Source: CAD feature listing. Evaluate the final solid. Frame: model axes, mm. Coordinates: 2 decimals unless noted, no trailing zeros. Loops run counter-clockwise (first coordinate to the right, second up) from the corner with the lowest first, then second, coordinate; pieces in that order, holes last.
Item 1: Section query B-B, the plane z = -6.4. Return the cut outline in (x, y) (3 decimals), then the cut area to 3 significant figures.
Item 2: Line query: probe 1 along Z at (x, y) = (41.6, 2.45) (3 decimals); probe 2 along Z at (x, y) = (35.2, 0.8) (3 decimals); probe 3 along X at (y, z) = (2, 14.4) (3 decimals). Output: solid intervals per line, ascending.
Item 3: Pin query (flat end, axial travel): pin 1 Ø2.5 at (x, z) = (6.4, 35.2) entering from -Y. Return the tip coordinate at first contact, or that it passes through.
Item 4: Section query D-D, the plane y = 2.5. State how many separate pieces and enclosed holes the cut face has, then the cut area to 3 significant figures.
Item 5: Section query A-A, the plane x = 20.8. Return the cut outline in (y, z) (3 decimals).
Item 6: Section query C-C, the plane x = 6.4. Return the cut outline in (y, z) (3 decimals), then the cut area to 3 significant figures.
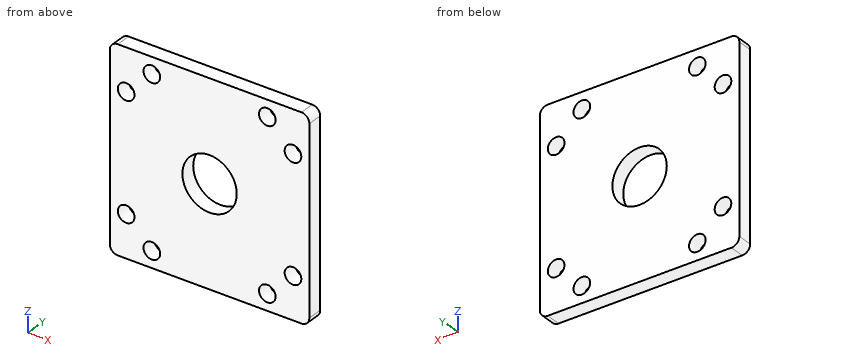
Autodesk Inventor part; units mm, degrees
ref_plane "YZ Plane" through (0, 0, 0) normal (1, 0, 0) x (0, 1, 0)
ref_plane "XZ Plane" through (0, 0, 0) normal (0, 1, 0) x (-1, 0, 0)
ref_plane "XY Plane" through (0, 0, 0) normal (0, 0, 1) x (1, 0, 0)
sketch "Sketch1" plane through (0, 0, 0) normal (0, 1, 0) x (-1, 0, 0)
  circle A0 centre (-20.8, 14.4) radius 6.7838
  circle A1 centre (-42.7, -7.5) radius 1.875
  circle A2 centre (1.1, 36.3) radius 1.875
  circle A3 centre (1.1, -7.5) radius 1.875
  circle A4 centre (-42.7, 36.3) radius 1.875
  circle A5 centre (-6.4, 35.2) radius 2.0734
  circle A6 centre (-35.2, -6.4) radius 2.0734
  circle A7 centre (-6.4, -6.4) radius 2.0734
  circle A8 centre (0, 0) radius 2.0734
  line L0 (-37.85, 31.45) -> (-37.85, -2.65)
  line L1 (-3.75, 31.45) -> (-37.85, 31.45)
  line L2 (-3.75, -2.65) -> (-3.75, 31.45)
  line L3 (-37.85, -2.65) -> (-3.75, -2.65)
  circle A9 centre (0, 28.8) radius 2.0734
  circle A10 centre (-35.2, 35.2) radius 2.0734
  circle A11 centre (-41.6, 0) radius 2.0734
  circle A12 centre (-41.6, 28.8) radius 2.0734
  line L4 (-43.7, 39.275) -> (2.1, 39.275)
  arc A13 (-43.7, 39.275) -> (-45.675, 37.3) centre (-43.7, 37.3) ccw
  line L5 (-45.675, -8.5) -> (-45.675, 37.3)
  arc A14 (-45.675, -8.5) -> (-43.7, -10.475) centre (-43.7, -8.5) ccw
  line L6 (2.1, -10.475) -> (-43.7, -10.475)
  arc A15 (2.1, -10.475) -> (4.075, -8.5) centre (2.1, -8.5) ccw
  line L7 (4.075, 37.3) -> (4.075, -8.5)
  arc A16 (4.075, 37.3) -> (2.1, 39.275) centre (2.1, 37.3) ccw
  line L8 (-3.75, 14.4) -> (-37.85, 14.4)
  dimension "d36" = 13.5675
extrude "Extrusion1" add sketch "Sketch1" along normal blind 3.75 contours L8 L2 L3 L0 A0 | A0 L8 L0 L1 L2 | A1 | A2 | A3 | A4 | L4 A16 L7 A15 L6 A14 L5 A13
properties part number "Top Mount (SM05)"
Verdict:
1. outline: (-4.075, 0) - (4.327, 0) - (4.327, 3.75) - (-4.075, 3.75) - close; (8.473, 0) - (33.127, 0) - (33.127, 3.75) - (8.473, 3.75) - close; (37.273, 0) - (45.675, 0) - (45.675, 3.75) - (37.273, 3.75) - close
1. area: 155 mm2
2. probe 1: z = -10.475 to -2.073, 2.073 to 26.727, 30.873 to 39.275
2. probe 2: z = -10.475 to -8.473, -4.327 to 33.127, 37.273 to 39.275
2. probe 3: x = -4.075 to 14.016, 27.584 to 45.675
3. pin 1: passes through
4. separate pieces: 1
4. enclosed holes: 9
4. area: 2,220 mm2
5. outline: (0, -10.475) - (3.75, -10.475) - (3.75, 7.616) - (0, 7.616) - close; (0, 21.184) - (3.75, 21.184) - (3.75, 39.275) - (0, 39.275) - close
6. outline: (0, -10.475) - (3.75, -10.475) - (3.75, -8.473) - (0, -8.473) - close; (0, -4.327) - (3.75, -4.327) - (3.75, 33.127) - (0, 33.127) - close; (0, 37.273) - (3.75, 37.273) - (3.75, 39.275) - (0, 39.275) - close
6. area: 155 mm2
